Build history of the part. All positions in model axes, mm. Give positions to 0.01 mm unless a question says otherwise; leave off trailing zeros. Order: outer loops, then holes, each group sorted by start corner. A loop starts at its lowest first (then second) coordinate and runs counter-clockwise, first axis right, second up. Notation, with made-up numbers: (-13.75, -28.5) -> (4.25, -28.5) arc R25 cw to (4.25, -9.5) -> close; hole circle Ø7 at (37.25, 69.5). An arc over 180 degrees is marked (long way). One line per item, written item: value. Start each with the question number.
(1) Probe line 1 (Y direction, x = 44.45, z = 0.25); line 2 (X direction, y = 35.5, z = -3.75); line 3 (X direction, y = 44.45, z = -3). List the from-to ranges inside material, lowest first.
(2) Saw through at A-A on y = 6.35. Give the cut face in (x, z).
(3) Saw through at C-C on z = -1.5. Give the cut face in (x, y).
(4) Pin check, flat tip, straight feed: pin 1 (6.5 mm diameter, centred on x = 44.45, y = 6.35, fed in from +Z). Stop position of the tip, or through.
(5) Saw through at D-D on x = 35.56. Give the cut face in (y, z), plus the area to 3 significant figures.
(6) Two-plate mould, pull along Z, no slides. Class faces 1 (the flat face through (25, 26, 6.35)), 2 (the cylindrical face through (23.397, 25.756, 0.631)), 3 (the cylindrical face through (5.201, 4.142, -1.637)): +Z half, -Z half, draft (parallel to the pull), parting line (faces both ways), or undercut.
(7) Saw through at B-B on x = 44.45. Give the cut face in (y, z).
```python
from build123d import *

# Parameters (mm, degrees)
F0_W           = 50.8
F0_H           = 50.8
F1_DEPTH       = 6.35
F1_DEPTH_BACK  = 6.35
F3_D           = 8.4
F5_D           = 4.9784
F5_CSINK_D     = 10.4394
F5_CSINK_ANGLE = 82
F6_D           = 4.2


with BuildPart() as f1:
    # F0 (on Top) → F1 (new body, two sides)
    with BuildSketch(Plane.XY) as f1_sk:
        with Locations((25.4, 25.4)):
            Rectangle(F0_W, F0_H)
    extrude(amount=-F1_DEPTH)
    extrude(f1_sk.sketch, amount=F1_DEPTH_BACK)

    # F3 (through all)
    with Locations(Plane.XZ):
        with Locations((15.24, 0), (35.56, 0)):
            Hole(F3_D / 2)

    # F5 (through all)
    with Locations(Plane.XY.offset(6.35)):
        with Locations((6.35, 44.45), (6.35, 6.35), (44.45, 6.35), (44.45, 44.45)):
            CounterSinkHole(F5_D / 2, F5_CSINK_D / 2, counter_sink_angle=F5_CSINK_ANGLE)

    # F6 (through all)
    with Locations(Plane.XZ):
        with Locations((25.4, 0)):
            Hole(F6_D / 2)


solid = f1.part
```
Results below:
1. line 1: y = 0 to 3.86, 8.84 to 41.96, 46.94 to 50.8
1. line 2: x = 0 to 13.35, 17.13 to 33.67, 37.45 to 50.8
1. line 3: x = 0 to 3.86, 8.84 to 12.3, 18.18 to 32.62, 38.5 to 41.96, 46.94 to 50.8
2. outline: (0, -6.35) -> (3.86, -6.35) -> (3.86, 3.21) -> (1.13, 6.35) -> (0, 6.35) -> close; (8.84, -6.35) -> (41.96, -6.35) -> (41.96, 3.21) -> (39.23, 6.35) -> (11.57, 6.35) -> (8.84, 3.21) -> close; (46.94, -6.35) -> (50.8, -6.35) -> (50.8, 6.35) -> (49.67, 6.35) -> (46.94, 3.21) -> close; hole circle Ø8.4 at (15.24, 0); hole circle Ø4.2 at (25.4, 0); hole circle Ø8.4 at (35.56, 0)
3. outline: (0, 0) -> (11.32, 0) -> (11.32, 50.8) -> (0, 50.8) -> close; (19.16, 0) -> (23.93, 0) -> (23.93, 50.8) -> (19.16, 50.8) -> close; (26.87, 0) -> (31.64, 0) -> (31.64, 50.8) -> (26.87, 50.8) -> close; (39.48, 0) -> (50.8, 0) -> (50.8, 50.8) -> (39.48, 50.8) -> close; hole circle Ø4.98 at (6.35, 6.35); hole circle Ø4.98 at (6.35, 44.45); hole circle Ø4.98 at (44.45, 6.35); hole circle Ø4.98 at (44.45, 44.45)
4. pin 1: stops at z = 4.08
5. outline: (0, -6.35) -> (50.8, -6.35) -> (50.8, -4.2) -> (0, -4.2) -> close; (0, 4.2) -> (50.8, 4.2) -> (50.8, 6.35) -> (0, 6.35) -> close
5. area: 218 mm²
6. face 1: +Z half
6. face 2: undercut
6. face 3: draft
7. outline: (0, -6.35) -> (3.86, -6.35) -> (3.86, 3.21) -> (1.13, 6.35) -> (0, 6.35) -> close; (8.84, -6.35) -> (41.96, -6.35) -> (41.96, 3.21) -> (39.23, 6.35) -> (11.57, 6.35) -> (8.84, 3.21) -> close; (46.94, -6.35) -> (50.8, -6.35) -> (50.8, 6.35) -> (49.67, 6.35) -> (46.94, 3.21) -> close
